The listing builds one solid part. Answer for the finished solid, in the listing's coordinates (mm). Face numbers are marked on the shaded views. A direction names the side the tool comes from. Give positions to 0.01 mm unless a question says otherwise; leave off trailing zeros. Loops run counter-clockwise (first coordinate to the right, second up) from the corner with the lowest first, then second, coordinate; pieces in that order, holes last. Notation, with made-up numbers: M 37,33 L 69,33 A19 cw 69,39 Z; hole C 89,-30 d6. An arc over 180 degrees is marked long. One line per item, written item: value. Start each with the question number.
Q1. Flat-ended cylindrical pins translate along their axes: pin 1 (3 mm diameter, centred on x = -20, z = -1, fed in from -Y); pin 2 (1.2 mm diameter, centred on x = -22.5, y = -16.5, fed in from +Z); pin 3 (6 mm diameter, centred on x = 2.5, z = -4, fed in from -Y); pin 4 (3 mm diameter, centred on x = 20.5, z = -2.5, fed in from -Y). Find the tip coordinate at first contact, or state that the pin passes through.
Q2. Consider L1, parallel to X at y = 1, z = 0; L2, parallel to X at y = -23.5, z = 1.5; L3, parallel to Y at x = -1, z = 15.5. Determine where each line is inside the solid, lowest interval first.
Q3. For the marked faces 1, 2, 3 and 4, determine the directions among +Z, -Z, +X, -X, +Y, -Y from which every point of the face is accessible in a straight line to the end or side of a thin tool.
Q4. A cutting plane is placed at A-A, the plane x = -21. Determine the outline of the cut face in (y, z), and give its area (3 significant figures).
Q5. A cutting plane is placed at D-D, the plane x = -8.5. Determine the outline of the cut face in (y, z).
Q6. A cutting plane is placed at C-C, the plane x = 2. Determine the outline of the cut face in (y, z).
Q7. The mould has two halves that part along X. Classify the marked faces 5, 6 and 7: +X half, -X half, draft (parallel to the pull), parting line (faces both ways), or undercut.
Q8. A cutting plane is placed at B-B, the plane z = 0. Determine the outline of the cut face in (x, y), and give its area (3 significant figures).
from build123d import *
from OCP.BRepFilletAPI import BRepFilletAPI_MakeChamfer

# Parameters (mm, degrees)
DODANIE_WYCI_GNI_CIE2_DEPTH = 2.5
SZKIC6_R                    = 3.6
WYTNIJ_WYCI_GNI_CIE3_DEPTH  = 37.881567212
DODANIE_WYCI_GNI_CIE3_DEPTH = 20
DODANIE_WYCI_GNI_CIE4_DEPTH = 10
ZAOKR_GLENIE1_R             = 1
ZAOKR_GLENIE2_R             = 5
WYTNIJ_WYCI_GNI_CIE1_REACH  = 59.319
SZKIC3_W                    = 18
SZKIC3_H                    = 2.5
SFAZOWANIE1_SIZE            = 1.2
SFAZOWANIE1_SIZE2           = 2.078460969
ZAOKR_GLENIE4_R             = 2
LUSTRO1_START               = -16
LUSTRO1_DEPTH               = 16
LUSTRO1_START_2             = -30
LUSTRO1_2_DEPTH             = 13.578460969
LUSTRO1_START_3             = -22
LUSTRO1_3_DEPTH             = 5.578460969
LUSTRO1_START_4             = -18.183542828
LUSTRO1_4_DEPTH             = 2.183542828
LUSTRO1_START_5             = -12.281593534
LUSTRO1_5_DEPTH             = 24.563187068
LUSTRO1_START_6             = -26
LUSTRO1_6_DEPTH             = 10.3
WYTNIJ_WYCI_GNI_CIE2_REACH  = 51.094
SFAZOWANIE2_SIZE            = 1
ZAOKR_GLENIE3_R             = 3


with BuildPart() as part:
    # Szkic1 → Dodanie-wyciągnięcie2 (new body)
    with BuildSketch(Plane(origin=(0, 0, 0), x_dir=(1, 0, 0), z_dir=(0, 1, 0))):
        Polygon((-25, -11), (-25, -26), (25, -26), (25, -11), (25, 27), (-25, 27), align=None)
    extrude(amount=DODANIE_WYCI_GNI_CIE2_DEPTH)

    # Szkic6 → Wytnij-wyciągnięcie3 (cut, through all)
    with BuildSketch(Plane(origin=(0, 2.5, 0), x_dir=(1, 0, 0), z_dir=(0, 1, 0))):
        with Locations(Location((0, 0, 0), (0, 0, 270))):
            Circle(SZKIC6_R)
        with BuildLine():
            Line((7.778174593, 12.02081528), (13.435028843, 17.67766953))
            ThreePointArc((13.435028843, 17.67766953), (17.67766953, 17.67766953), (17.67766953, 13.435028843))
            Line((17.67766953, 13.435028843), (12.02081528, 7.778174593))
            ThreePointArc((12.02081528, 7.778174593), (7.778174593, 7.778174593), (7.778174593, 12.02081528))
        make_face()
        with BuildLine():
            Line((12.02081528, -7.778174593), (17.67766953, -13.435028843))
            ThreePointArc((17.67766953, -13.435028843), (17.67766953, -17.67766953), (13.435028843, -17.67766953))
            Line((13.435028843, -17.67766953), (7.778174593, -12.02081528))
            ThreePointArc((7.778174593, -12.02081528), (7.778174593, -7.778174593), (12.02081528, -7.778174593))
        make_face()
        with BuildLine():
            Line((-7.778174593, -12.02081528), (-13.435028843, -17.67766953))
            ThreePointArc((-13.435028843, -17.67766953), (-17.67766953, -17.67766953), (-17.67766953, -13.435028843))
            Line((-17.67766953, -13.435028843), (-12.02081528, -7.778174593))
            ThreePointArc((-12.02081528, -7.778174593), (-7.778174593, -7.778174593), (-7.778174593, -12.02081528))
        make_face()
        with BuildLine():
            Line((-12.02081528, 7.778174593), (-17.67766953, 13.435028843))
            ThreePointArc((-17.67766953, 13.435028843), (-17.67766953, 17.67766953), (-13.435028843, 17.67766953))
            Line((-13.435028843, 17.67766953), (-7.778174593, 12.02081528))
            ThreePointArc((-7.778174593, 12.02081528), (-7.778174593, 7.778174593), (-12.02081528, 7.778174593))
        make_face()
    extrude(amount=-WYTNIJ_WYCI_GNI_CIE3_DEPTH, mode=Mode.SUBTRACT)

    # Szkic2 → Dodanie-wyciągnięcie3 (add)
    with BuildSketch(Plane.XZ):
        Polygon((15.7, -6.5), (15.7, 6.5), (25, 15.172390301), (25, -15.172390301), align=None)
    extrude(amount=DODANIE_WYCI_GNI_CIE3_DEPTH)

    # Szkic8 → Dodanie-wyciągnięcie4 (add)
    with BuildSketch(Plane.XZ.offset(20)):
        Polygon((25, 15.172390301), (25, -15.172390301), (21.9, -12.281593534), (21.9, 12.281593534), align=None)
    extrude(amount=DODANIE_WYCI_GNI_CIE4_DEPTH)

    # Zaokrąglenie1
    zaokr_glenie1_edges = [part.edges().sort_by_distance(p)[0] for p in [
        (25, -15, 15.172390301),
        (25, -15, -15.172390301),
    ]]
    fillet(zaokr_glenie1_edges, radius=ZAOKR_GLENIE1_R)

    # Zaokrąglenie2
    zaokr_glenie2_edges = [part.edges().sort_by_distance(p)[0] for p in [
        (15.7, -10, 6.5),
        (15.7, -10, -6.5),
    ]]
    fillet(zaokr_glenie2_edges, radius=ZAOKR_GLENIE2_R)

    # Szkic3 → Wytnij-wyciągnięcie1 (cut, up to next)
    with BuildSketch(Plane.ZY.offset(-15.7), mode=Mode.PRIVATE) as wytnij_wyci_gni_cie1_sk1:
        with Locations((0, -17.25)):
            Rectangle(SZKIC3_W, SZKIC3_H)
    wytnij_wyci_gni_cie1_tool1 = extrude(wytnij_wyci_gni_cie1_sk1.sketch, amount=-WYTNIJ_WYCI_GNI_CIE1_REACH, mode=Mode.PRIVATE) & part.part
    add(wytnij_wyci_gni_cie1_tool1.solids().sort_by_distance((15.7, -17.25, 0))[0], mode=Mode.SUBTRACT)

    # Sfazowanie1: one chamfer whose edges measure the first distance from different faces: ONE call of the kernel's chamfer builder (chamfer() names one face for all edges)
    sfazowanie1_edges_1 = [part.edges().sort_by_distance(p)[0] for p in [
        (21.690460888, -18.5, -9),
    ]]
    sfazowanie1_side_1 = [part.faces().sort_by_distance(p)[0] for p in [
        (21.690460888, -17.25, -9),
    ]]
    sfazowanie1_edges_2 = [part.edges().sort_by_distance(p)[0] for p in [
        (21.690460888, -18.5, 9),
    ]]
    sfazowanie1_side_2 = [part.faces().sort_by_distance(p)[0] for p in [
        (21.690460888, -17.25, 9),
    ]]
    sfazowanie1 = BRepFilletAPI_MakeChamfer(part.part.solid().wrapped)
    for e in sfazowanie1_edges_1:
        sfazowanie1.Add(SFAZOWANIE1_SIZE, SFAZOWANIE1_SIZE2, e.wrapped, sfazowanie1_side_1[0].wrapped)  # the first distance lies on this face
    for e in sfazowanie1_edges_2:
        sfazowanie1.Add(SFAZOWANIE1_SIZE, SFAZOWANIE1_SIZE2, e.wrapped, sfazowanie1_side_2[0].wrapped)  # the first distance lies on this face
    add(Compound.cast(sfazowanie1.Shape()), mode=Mode.REPLACE)

    # Zaokrąglenie4
    zaokr_glenie4_edges = [part.edges().sort_by_distance(p)[0] for p in [
        (21.9, -20, 0),
    ]]
    fillet(zaokr_glenie4_edges, radius=ZAOKR_GLENIE4_R)

    # Lustro1: read off the stored shape, not the designer's step
    # Lustro1 outline → Lustro1 (add)
    with BuildSketch(Plane(origin=(0, 0, 0), x_dir=(1, 0, 0), z_dir=(0, 1, 0)).offset(LUSTRO1_START)):
        with BuildLine():
            ThreePointArc((-25, -12.872547754), (-24.398749069, -13.789607828), (-23.31800164, -13.603901455))
            Line((-23.31800164, -13.603901455), (-17.2900082, -7.982706633))
            ThreePointArc((-17.2900082, -7.982706633), (-16.114699628, -6.31968347), (-15.7, -4.325938125))
            Line((-15.7, -4.325938125), (-15.7, 4.325938125))
            ThreePointArc((-15.7, 4.325938125), (-16.114699628, 6.31968347), (-17.2900082, 7.982706633))
            Line((-17.2900082, 7.982706633), (-23.31800164, 13.603901455))
            ThreePointArc((-23.31800164, 13.603901455), (-24.398749069, 13.789607828), (-25, 12.872547754))
            Line((-25, 12.872547754), (-25, -12.872547754))
        make_face()
    extrude(amount=LUSTRO1_DEPTH)



with BuildPart() as body_2:
    # Lustro1 2 outline → Lustro1 2 (new body)
    with BuildSketch(Plane(origin=(0, 0, 0), x_dir=(1, 0, 0), z_dir=(0, 1, 0)).offset(LUSTRO1_START_2)):
        with BuildLine():
            ThreePointArc((-25, -12.872547754), (-24.398749069, -13.789607828), (-23.31800164, -13.603901455))
            Line((-23.31800164, -13.603901455), (-21.9, -12.281593534))
            Line((-21.9, -12.281593534), (-21.9, 12.281593534))
            Line((-21.9, 12.281593534), (-23.31800164, 13.603901455))
            ThreePointArc((-23.31800164, 13.603901455), (-24.398749069, 13.789607828), (-25, 12.872547754))
            Line((-25, 12.872547754), (-25, -12.872547754))
        make_face()
    extrude(amount=LUSTRO1_2_DEPTH)

    # Lustro1 3 outline → Lustro1 3 (add)
    with BuildSketch(Plane(origin=(0, 0, 0), x_dir=(1, 0, 0), z_dir=(0, 1, 0)).offset(LUSTRO1_START_3)):
        with BuildLine():
            Line((-21.9, -12.281593534), (-17.2900082, -7.982706633))
            ThreePointArc((-17.2900082, -7.982706633), (-16.114699628, -6.31968347), (-15.7, -4.325938125))
            Line((-15.7, -4.325938125), (-15.7, 4.325938125))
            ThreePointArc((-15.7, 4.325938125), (-16.114699628, 6.31968347), (-17.2900082, 7.982706633))
            Line((-17.2900082, 7.982706633), (-21.9, 12.281593534))
            Line((-21.9, 12.281593534), (-21.9, -12.281593534))
        make_face()
    extrude(amount=LUSTRO1_3_DEPTH)


with BuildPart() as part_1:
    add(part.part)

    add(body_2.part)  # Lustro1 4 merges body 2
    # Lustro1 4 outline → Lustro1 4 (add)
    with BuildSketch(Plane(origin=(0, 0, 0), x_dir=(1, 0, 0), z_dir=(0, 1, 0)).offset(LUSTRO1_START_4)):
        with BuildLine():
            Line((-25, -9), (-25, -12.872547754))
            ThreePointArc((-25, -12.872547754), (-24.398749069, -13.789607828), (-23.31800164, -13.603901455))
            Line((-23.31800164, -13.603901455), (-18.380921775, -9))
            Line((-18.380921775, -9), (-25, -9))
        make_face()
        with BuildLine():
            Line((-25, 12.872547754), (-25, 9))
            Line((-25, 9), (-18.380921775, 9))
            Line((-18.380921775, 9), (-23.31800164, 13.603901455))
            ThreePointArc((-23.31800164, 13.603901455), (-24.398749069, 13.789607828), (-25, 12.872547754))
        make_face()
    extrude(amount=LUSTRO1_4_DEPTH)

    # Lustro1 5 outline → Lustro1 5 (cut)
    with BuildSketch(Plane.XY.offset(LUSTRO1_START_5)):
        with BuildLine():
            Line((-15.7, -22), (-15.7, -20))
            Line((-15.7, -20), (-19.9, -20))
            ThreePointArc((-19.9, -20), (-21.314213562, -20.585786438), (-21.9, -22))
            Line((-21.9, -22), (-15.7, -22))
        make_face()
    extrude(amount=LUSTRO1_5_DEPTH, mode=Mode.SUBTRACT)

    # Lustro1 6 outline → Lustro1 6 (cut)
    with BuildSketch(Plane.YZ.offset(LUSTRO1_START_6)):
        Polygon((-18.5, 7.8), (-18.5, -7.8), (-16.421539031, -9), (-16.421539031, 9), align=None)
    extrude(amount=LUSTRO1_6_DEPTH, mode=Mode.SUBTRACT)

    # Szkic5 → Wytnij-wyciągnięcie2 (cut, up to next)
    with BuildSketch(Plane(origin=(0, 2.5, 0), x_dir=(1, 0, 0), z_dir=(0, 1, 0)), mode=Mode.PRIVATE) as wytnij_wyci_gni_cie2_sk1:
        with BuildLine():
            Line((22.55, 21), (22.55, 18))
            ThreePointArc((22.55, 18), (21, 16.45), (19.45, 18))
            Line((19.45, 18), (19.45, 21))
            ThreePointArc((19.45, 21), (21, 22.55), (22.55, 21))
        make_face()
    wytnij_wyci_gni_cie2_tool1 = extrude(wytnij_wyci_gni_cie2_sk1.sketch, amount=-WYTNIJ_WYCI_GNI_CIE2_REACH, mode=Mode.PRIVATE) & part_1.part
    wytnij_wyci_gni_cie2 = wytnij_wyci_gni_cie2_tool1.solids().sort_by_distance((21, 2.5, -19.5))[0]
    add(wytnij_wyci_gni_cie2, mode=Mode.SUBTRACT)

    # Lustro2: Wytnij-wyciągnięcie2 across plane
    add(wytnij_wyci_gni_cie2.mirror(Plane(origin=(0, 0, 0), x_dir=(0, 0, 1), z_dir=(1, 0, 0))), mode=Mode.SUBTRACT)

    # Sfazowanie2
    sfazowanie2_edges = [part_1.edges().sort_by_distance(p)[0] for p in [
        (25, -18.5, 0),
        (25, -17.9, -7.960769515),
        (25, -17.9, 7.960769515),
        (-25, -18.5, 0),
        (-25, -17.460769515, -8.4),
        (-25, -17.460769515, 8.4),
    ]]
    chamfer(sfazowanie2_edges, length=SFAZOWANIE2_SIZE)

    # Zaokrąglenie3
    zaokr_glenie3_edges = [part_1.edges().sort_by_distance(p)[0] for p in [
        (-25, 1.25, -27),
        (25, 1.25, -27),
    ]]
    fillet(zaokr_glenie3_edges, radius=ZAOKR_GLENIE3_R)


solid = part_1.part
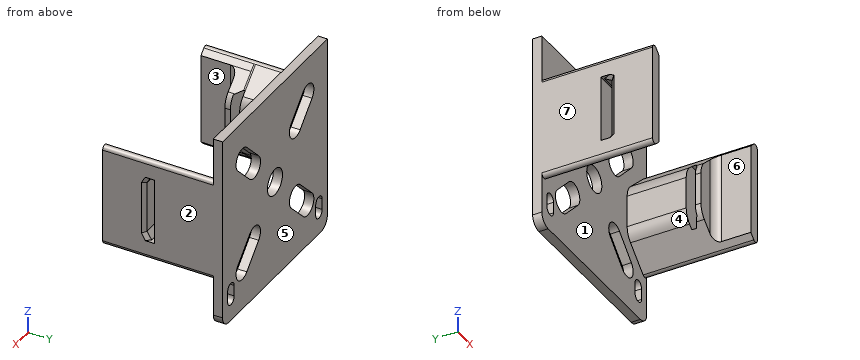
Answer block:
1. pin 1: y = -20.8
1. pin 2: z = 13.4
1. pin 3: y = 0
1. pin 4: y = -30
2. L1: -25 to -3.6, 3.6 to 25
2. L2: -25 to -21.9, 21.9 to 25
2. L3: 0 to 2.5
3. face 1: -Y
3. face 2: +Z, -Z, +X, +Y, -Y
3. face 3: +Z, -Z, -Y
3. face 4: -Z, -Y
4. outline: M -20.33,-11.44 L 0,-11.44 L 0,-16.45 L 2.5,-16.45 L 2.5,26 L 0,26 L 0,11.44 L -20.33,11.44 Z; M 0,-27 L 2.5,-27 L 2.5,-22.55 L 0,-22.55 Z; hole M -18.5,-7.8 L -16.42,-9 L -16,-9 L -16,9 L -16.42,9 L -18.5,7.8 Z
4. area: 540 mm^2
5. outline: M 0,-27 L 2.5,-27 L 2.5,-12.74 L 0,-12.74 Z; M 0,-7.25 L 2.5,-7.25 L 2.5,7.25 L 0,7.25 Z; M 0,12.74 L 2.5,12.74 L 2.5,26 L 0,26 Z
6. outline: M 0,-27 L 2.5,-27 L 2.5,-2.99 L 0,-2.99 Z; M 0,2.99 L 2.5,2.99 L 2.5,26 L 0,26 Z
7. face 5: draft
7. face 6: undercut
7. face 7: -X half
8. outline: M -25,-30 L -21.9,-30 L -21.9,-22 A2 cw -19.9,-20 L -15.7,-20 L -15.7,-18.5 L -24,-18.5 L -25,-19.5 Z; M -25,-16 L -15.7,-16 L -15.7,0 L -3.6,0 L -3.6,2.5 L -25,2.5 Z; M 3.6,0 L 15.7,0 L 15.7,-16 L 25,-16 L 25,2.5 L 3.6,2.5 Z; M 15.7,-20 L 19.9,-20 A2 cw 21.9,-22 L 21.9,-30 L 25,-30 L 25,-19.5 L 24,-18.5 L 15.7,-18.5 Z
8. area: 495 mm^2
